The model under review builds one solid part; all positions refer to its coordinate system, in mm. A direction names the side the tool comes from. Give positions to 0.01 mm unless a question says otherwise; leave off trailing zeros. Order: outer loops, then holes, each group sorted by start corner. A loop starts at its lowest first (then second) coordinate and runs counter-clockwise, first axis right, second up.
```python
from build123d import *

# Parameters (mm, degrees)
CYLINDER006_R          = 14
CYLINDER006_DEPTH      = 3
CYLINDER006_ROLL_ANGLE = -90
CYLINDER005_R          = 14
CYLINDER005_DEPTH      = 3
CYLINDER005_ROLL_ANGLE = -90
CYLINDER004_R          = 2.3
CYLINDER004_DEPTH      = 40
CYLINDER003_R          = 2
CYLINDER003_DEPTH      = 40
CYLINDER002_R          = 2.3
CYLINDER002_DEPTH      = 40
CYLINDER001_R          = 2.3
CYLINDER001_DEPTH      = 40
BOX005_W               = 1
BOX005_H               = 85
BOX005_DEPTH           = 23.5
BOX004_W               = 1
BOX004_H               = 85
BOX004_DEPTH           = 23.5
BOX003_W               = 10
BOX003_H               = 90
BOX003_DEPTH           = 10
BOX003_ROLL_ANGLE      = 3e-06
BOX003_PITCH_ANGLE     = -44.999934
BOX003_PLACEMENT_ANGLE = -7e-06
BOX002_W               = 10
BOX002_H               = 90
BOX002_DEPTH           = 10
BOX002_ROLL_ANGLE      = 3e-06
BOX002_PITCH_ANGLE     = 44.999934
BOX002_PLACEMENT_ANGLE = 7e-06
BOX001_W               = 25
BOX001_H               = 85
BOX001_DEPTH           = 6
CYLINDER_R             = 8.1
CYLINDER_DEPTH         = 100
CYLINDER_ROLL_ANGLE    = -90
BOX_W                  = 50
BOX_H                  = 85
BOX_DEPTH              = 32.5


with BuildPart() as cylinder006:
    # Cylinder006 → Cylinder006 (new body)
    with BuildSketch(Plane.XY):
        Circle(CYLINDER006_R)
    extrude(amount=CYLINDER006_DEPTH)


with BuildPart() as cylinder006_1:
    # Cylinder006 roll: moved
    add(cylinder006.part.rotate(Axis((0, 0, 0), (1, 0, 0)), CYLINDER006_ROLL_ANGLE))


with BuildPart() as cylinder006_2:
    # Cylinder006 placement: moved
    add(cylinder006_1.part.moved(Location((25.6346, 83, 19.0294))))


with BuildPart() as cylinder005:
    # Cylinder005 → Cylinder005 (new body)
    with BuildSketch(Plane.XY):
        Circle(CYLINDER005_R)
    extrude(amount=CYLINDER005_DEPTH)


with BuildPart() as cylinder005_1:
    # Cylinder005 roll: moved
    add(cylinder005.part.rotate(Axis((0, 0, 0), (1, 0, 0)), CYLINDER005_ROLL_ANGLE))


with BuildPart() as cylinder005_2:
    # Cylinder005 placement: moved
    add(cylinder005_1.part.moved(Location((25.5737, -1, 19.0038))))


with BuildPart() as cylinder004:
    # Cylinder004 → Cylinder004 (new body)
    with BuildSketch(Plane(origin=(43, 72.5, -4), x_dir=(1, 0, 0), z_dir=(0, 0, 1))):
        Circle(CYLINDER004_R)
    extrude(amount=CYLINDER004_DEPTH)


with BuildPart() as cylinder003:
    # Cylinder003 → Cylinder003 (new body)
    with BuildSketch(Plane(origin=(43, 12.5, -4), x_dir=(1, 0, 0), z_dir=(0, 0, 1))):
        Circle(CYLINDER003_R)
    extrude(amount=CYLINDER003_DEPTH)


with BuildPart() as cylinder002:
    # Cylinder002 → Cylinder002 (new body)
    with BuildSketch(Plane(origin=(7, 72.5, -3), x_dir=(1, 0, 0), z_dir=(0, 0, 1))):
        Circle(CYLINDER002_R)
    extrude(amount=CYLINDER002_DEPTH)


with BuildPart() as cylinder001:
    # Cylinder001 → Cylinder001 (new body)
    with BuildSketch(Plane(origin=(7, 12.5, -2), x_dir=(1, 0, 0), z_dir=(0, 0, 1))):
        Circle(CYLINDER001_R)
    extrude(amount=CYLINDER001_DEPTH)


with BuildPart() as box005:
    # Box005 → Box005 (new body)
    with BuildSketch(Plane(origin=(49, 0, 9), x_dir=(1, 0, 0), z_dir=(0, 0, 1))):
        with Locations((0.5, 42.5)):
            Rectangle(BOX005_W, BOX005_H)
    extrude(amount=BOX005_DEPTH)


with BuildPart() as box004:
    # Box004 → Box004 (new body)
    with BuildSketch(Plane.XY.offset(9)):
        with Locations((0.5, 42.5)):
            Rectangle(BOX004_W, BOX004_H)
    extrude(amount=BOX004_DEPTH)


with BuildPart() as box003:
    # Box003 → Box003 (new body)
    with BuildSketch(Plane.XY):
        with Locations((5, 45)):
            Rectangle(BOX003_W, BOX003_H)
    extrude(amount=BOX003_DEPTH)


with BuildPart() as box003_1:
    # Box003 roll: moved
    add(box003.part.rotate(Axis((0, 0, 0), (1, 0, 0)), BOX003_ROLL_ANGLE))


with BuildPart() as box003_2:
    # Box003 pitch: moved
    add(box003_1.part.rotate(Axis((0, 0, 0), (0, 1, 0)), BOX003_PITCH_ANGLE))


with BuildPart() as box003_3:
    # Box003 placement: moved
    add(box003_2.part.moved(Location((-18.82, -2, 2.25))).rotate(Axis((-18.82, -2, 2.25), (0, 0, 1)), BOX003_PLACEMENT_ANGLE))


with BuildPart() as box002:
    # Box002 → Box002 (new body)
    with BuildSketch(Plane.XY):
        with Locations((5, 45)):
            Rectangle(BOX002_W, BOX002_H)
    extrude(amount=BOX002_DEPTH)


with BuildPart() as box002_1:
    # Box002 roll: moved
    add(box002.part.rotate(Axis((0, 0, 0), (1, 0, 0)), BOX002_ROLL_ANGLE))


with BuildPart() as box002_2:
    # Box002 pitch: moved
    add(box002_1.part.rotate(Axis((0, 0, 0), (0, 1, 0)), BOX002_PITCH_ANGLE))


with BuildPart() as box002_3:
    # Box002 placement: moved
    add(box002_2.part.moved(Location((-50.8986, -3, 9.31859))).rotate(Axis((-50.8986, -3, 9.31859), (0, 0, 1)), BOX002_PLACEMENT_ANGLE))


with BuildPart() as cut002:
    # Box001 → Box001 (new body)
    with BuildSketch(Plane(origin=(-43.825523, -3.3e-05, 2.247464), x_dir=(1, 0, 0), z_dir=(0, 0, 1))):
        with Locations((12.5, 42.5)):
            Rectangle(BOX001_W, BOX001_H)
    extrude(amount=BOX001_DEPTH)

    # Cut001: cut Box002
    add(box002_3.part, mode=Mode.SUBTRACT)

    # Cut002: cut Box003
    add(box003_3.part, mode=Mode.SUBTRACT)


with BuildPart() as cut002_1:
    # Cut002 placement: moved
    add(cut002.part.moved(Location((56.6969, -0.000184, 30.2))))


with BuildPart() as cylinder:
    # Cylinder → Cylinder (new body)
    with BuildSketch(Plane.XY):
        Circle(CYLINDER_R)
    extrude(amount=CYLINDER_DEPTH)


with BuildPart() as cylinder_1:
    # Cylinder roll: moved
    add(cylinder.part.rotate(Axis((0, 0, 0), (1, 0, 0)), CYLINDER_ROLL_ANGLE))


with BuildPart() as cylinder_2:
    # Cylinder placement: moved
    add(cylinder_1.part.moved(Location((25, -4.78696, 19))))


with BuildPart() as cut011:
    # Box → Box (new body)
    with BuildSketch(Plane.XY):
        with Locations((25, 42.5)):
            Rectangle(BOX_W, BOX_H)
    extrude(amount=BOX_DEPTH)

    # Cut: cut Cylinder
    add(cylinder_2.part, mode=Mode.SUBTRACT)

    # Fusion: union Cut002
    add(cut002_1.part)

    # Cut003: cut Box004
    add(box004.part, mode=Mode.SUBTRACT)

    # Cut004: cut Box005
    add(box005.part, mode=Mode.SUBTRACT)

    # Cut005: cut Cylinder001
    add(cylinder001.part, mode=Mode.SUBTRACT)

    # Cut006: cut Cylinder002
    add(cylinder002.part, mode=Mode.SUBTRACT)

    # Cut007: cut Cylinder003
    add(cylinder003.part, mode=Mode.SUBTRACT)

    # Cut008: cut Cylinder004
    add(cylinder004.part, mode=Mode.SUBTRACT)

    # Cut009: cut Cylinder005
    add(cylinder005_2.part, mode=Mode.SUBTRACT)

    # Cut010: cut Cylinder005
    add(cylinder005_2.part, mode=Mode.SUBTRACT)

    # Cut011: cut Cylinder006
    add(cylinder006_2.part, mode=Mode.SUBTRACT)


solid = cut011.part
```
1. Take a section at C-C (y = 12.5). Write out the cut boundary in (x, z).
2. For faces 4 (the cylindrical face through (22.54, 0.99, 32.67)), 5 (the flat face through (7, 43, 32.5)), 6 (the flat face through (49, 42, 21)), 7 (the flat face through (50, 42, 4)), list the 3-axis set-ups (+Z, -Z, +X, -X, +Y, -Y) from which the entire face can be reached by the end or side of a thin tool; tool diameter is ignored.
3. Take a section at D-D (y = 33.5). Write out the cut boundary in (x, z), and give its area (3 significant figures).
4. Take a section at B-B (x = 43). Write out the cut boundary in (y, z), and give its area (3 significant figures).
5. Insertion check: pin 1 (5 mm diameter, centred on y = 27, z = 19.5, fed in from +X); pin 2 (23 mm diameter, centred on x = 8, y = 25.5, fed in from +Z); pin 3 (6 mm diameter, centred on x = 39, y = 34, fed in from +Z); pin 4 (8.5 mm diameter, centred on x = 24.5, z = 12.5, fed in from -Y). Each pin has a flat end and moves straight along its axis. Give the tip position at first contact, or say it passes through.
6. Draft analysis for pull direction X (two halves, no side actions). For faces 1 (the flat face through (25, 43, 38.447)), 2 (the cylindrical face through (6.501, 70.255, 16.022)), 3 (the flat face through (1, 42, 21)), state which applies: pulls with the +X half, pulls with the -X half, needs draft (parallel to the pull), parting line crosses it, or undercut.
7. Take a section at A-A (y = 72.5). Write out the cut boundary in (x, z), and give its area (3 significant figures).
8. To check wall thickness, follow line 1 (Y direction, x = 43, z = 15); line 2 (X direction, y = 72.5, z = 12.5); line 3 (Y direction, x = 7, z = 21). State the ranges of each line that lie inside material, in increasing order.
Answer:
1. outline: (0, 0) - (4.7, 0) - (4.7, 32.5) - (1, 32.5) - (1, 9) - (0, 9) - close; (9.3, 0) - (41, 0) - (41, 32.5) - (37.83, 32.5) - (31.88, 38.45) - (18.87, 38.45) - (12.92, 32.5) - (9.3, 32.5) - close; (45, 0) - (50, 0) - (50, 9) - (49, 9) - (49, 32.5) - (45, 32.5) - close; hole circle Ø16.2 at (25, 19)
2. face 4: -Y
2. face 5: +Z, -X, +Y, -Y
2. face 6: +Z, +X, +Y, -Y
2. face 7: +Z, -Z, +X, +Y, -Y
3. outline: (0, 0) - (50, 0) - (50, 9) - (49, 9) - (49, 32.5) - (37.83, 32.5) - (31.88, 38.45) - (18.87, 38.45) - (12.92, 32.5) - (1, 32.5) - (1, 9) - (0, 9) - close; hole circle Ø16.2 at (25, 19)
3. area: 1,480 mm2
4. outline: (0, 0) - (10.5, 0) - (10.5, 32.5) - (0, 32.5) - close; (14.5, 0) - (70.2, 0) - (70.2, 32.5) - (14.5, 32.5) - close; (74.8, 0) - (85, 0) - (85, 32.5) - (74.8, 32.5) - close
4. area: 2,480 mm2
5. pin 1: stops at x = 49
5. pin 2: stops at z = 38.45
5. pin 3: stops at z = 34.33
5. pin 4: stops at y = 2
6. face 1: needs draft
6. face 2: undercut
6. face 3: pulls with the -X half
7. outline: (0, 0) - (4.7, 0) - (4.7, 32.5) - (1, 32.5) - (1, 9) - (0, 9) - close; (9.3, 0) - (40.7, 0) - (40.7, 32.5) - (37.83, 32.5) - (31.88, 38.45) - (18.87, 38.45) - (12.92, 32.5) - (9.3, 32.5) - close; (45.3, 0) - (50, 0) - (50, 9) - (49, 9) - (49, 32.5) - (45.3, 32.5) - close; hole circle Ø16.2 at (25, 19)
7. area: 1,190 mm2
8. line 1: y = 0 to 10.5, 14.5 to 70.2, 74.8 to 85
8. line 2: x = 1 to 4.7, 9.3 to 20.17, 29.83 to 40.7, 45.3 to 49
8. line 3: y = 0 to 10.2, 14.8 to 70.2, 74.8 to 85
